Answer from the drawing. Dimensions are ordinates in mm from the lowest x, y and z of the part. Give positions to 0.01 mm unless a question says otherwise; leave off trailing zeros. Write each loop counter-clockwise with the first axis right and the second up, starting at its lowest first coordinate (ties: lowest second). Pieces come first, ordered by that corner, then holes. Notation, with made-up numbers: M 69.5,-14 L 118.5,-14 A19 ccw 118.5,-3 Z; hole C 32,54.5 d1. An arc over 180 degrees is marked long. Write each question's results on one line, items separated by ' | '. Start each with the question number.
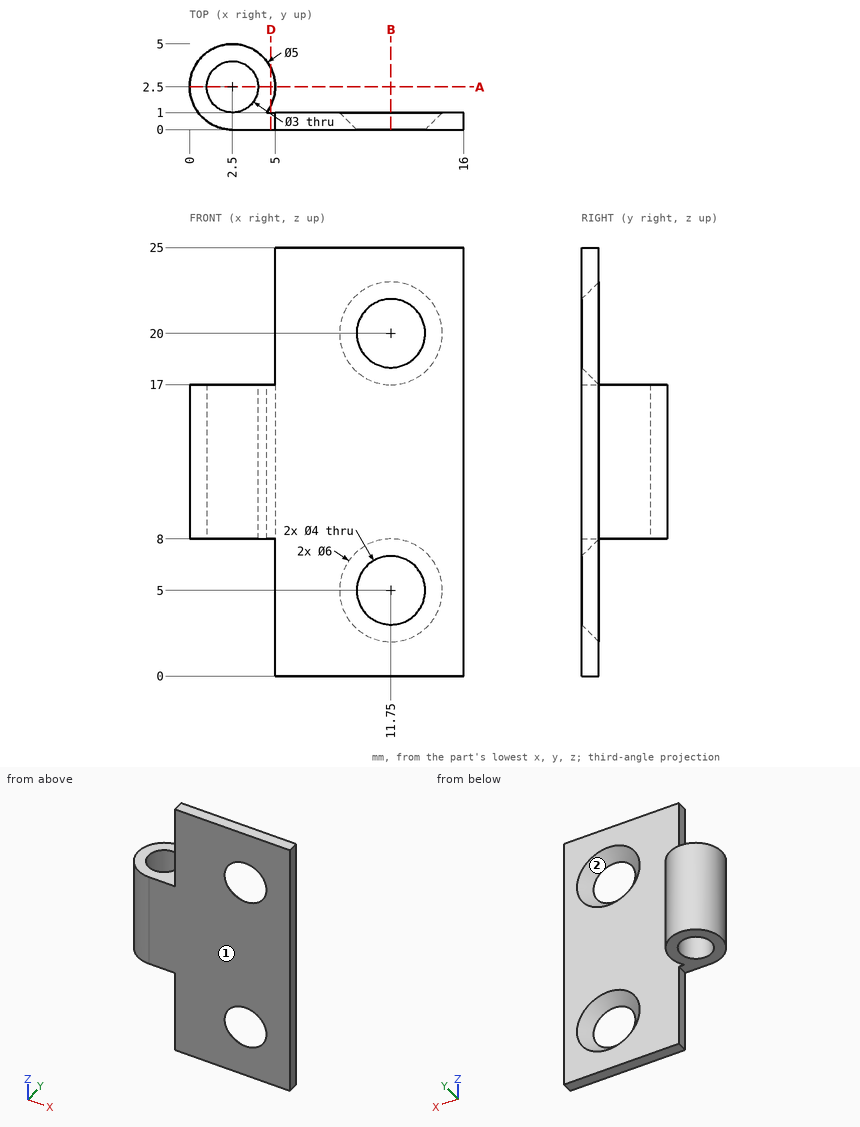
Item 1: Given P1, Ø5, axis at x = 6.5, z = 19, coming from the -Y side; P2, Ø3.5, axis at x = 11, z = 8, coming from the +Y side; P3, Ø0.8, axis at y = 0.5, z = 21.5, coming from the -X side; P4, Ø3.5, axis at x = 11.75, z = 5, coming from the +Y side, each flat-ended and moving along its own axis, determine where each tip first touches the part or whether it passes through.
Item 2: Determine the mould class of the marked faces 1 and 2 for opening direction X: +X half, -X half, draft (parallel to the pull), parting line (faces both ways), or undercut.
Item 3: Section D-D, the plane x = 4.75 is taken. Determine the outline of the cut face in (y, z).
Item 4: Section A-A, the plane y = 2.5 is taken. Determine the outline of the cut face in (x, z).
Item 5: Straight lines are drawn through the part: line 1 (X direction, y = 2.5, z = 14); line 2 (Z direction, x = 11.75, y = 0.05). For each, find the intervals that lie inside material, in ascending order.
Item 6: Section B-B, the plane x = 11.75 is taken. Give the number of separate pieces and of enclosed holes in the cut face, then the cut area to 3 significant figures.
Worked out:
1) P1: stops at y = 0 | P2: stops at y = 1 | P3: stops at x = 5 | P4: passes through
2) face 1: draft | face 2: undercut
3) outline: M 0,8 L 1,8 L 1,17 L 0,17 Z; M 1.41,8 L 3.59,8 L 3.59,17 L 1.41,17 Z
4) outline: M 0,8 L 1,8 L 1,17 L 0,17 Z; M 4,8 L 5,8 L 5,17 L 4,17 Z
5) line 1: x = 0 to 1, 4 to 5 | line 2: z = 0 to 2.95, 7.05 to 17.95, 22.05 to 25
6) separate pieces: 3 | enclosed holes: 0 | area: 15.0 mm²
